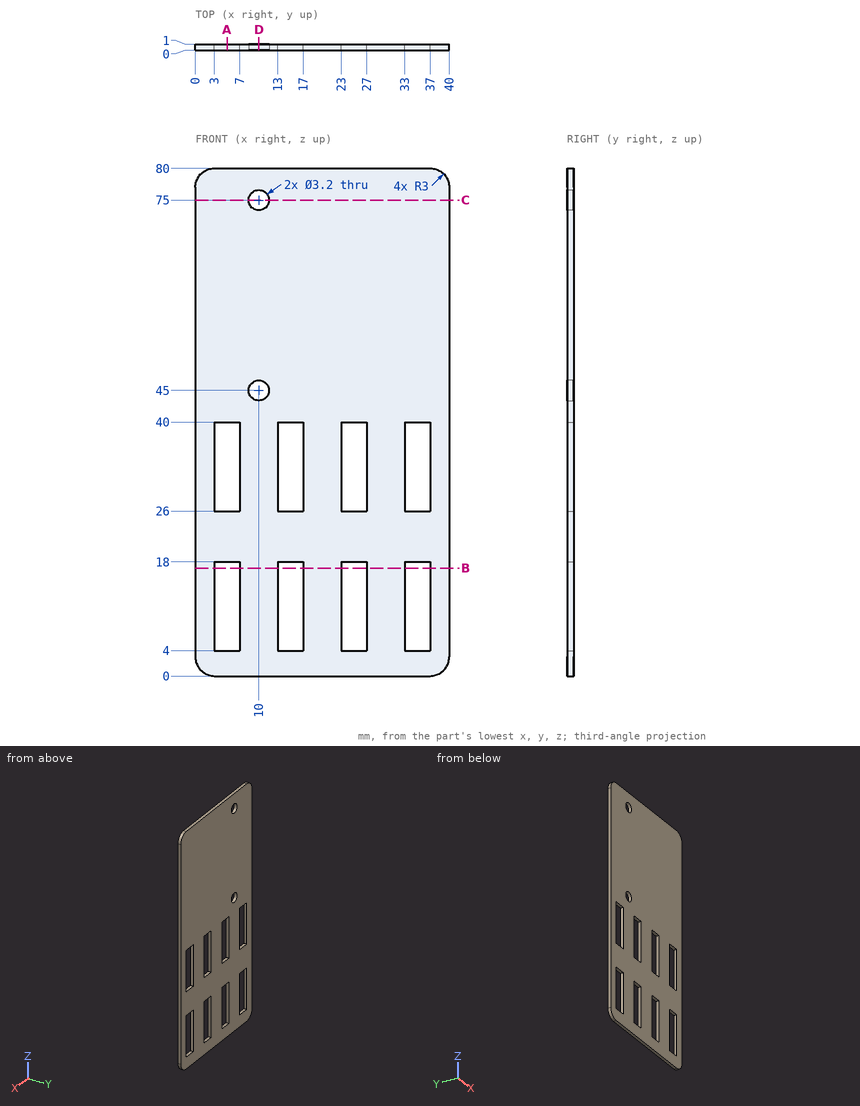
Drawing for the job (mm, zero at the part's lowest x, y, z). Coordinates: 2 decimals unless noted, no trailing zeros. Order: outer loops, then holes, each group sorted by start corner. A loop starts at its lowest first (then second) coordinate and runs counter-clockwise, first axis right, second up. Notation, with made-up numbers: (82, -11.75) -> (110, -11.75) arc R30 ccw to (110, 26.25) -> close; hole circle Ø1 at (26.25, 67.25). An arc over 180 degrees is marked (long way). Answer in a Markdown table with one row per item.
1) Flat gauge pin, fed straight in: P1, Ø3, axis at x = 10, z = 75, coming from the +Y side. Where does the tip first touch, or does it go through?
Check values:
| item | result |
|---|---|
| P1 | through |
2) Drill centre lines: line 1 (Z direction, x = 6, y = 0.4); line 2 (X direction, y = 0.7, z = 10); line 3 (X direction, y = 0.6, z = 75). Where is each one in solid material? Low to high.
Check values:
| item | result |
|---|---|
| line 1 | 0 to 4, 18 to 26, 40 to 80 |
| line 2 | 0 to 3, 7 to 13, 17 to 23, 27 to 33, 37 to 40 |
| line 3 | 0 to 8.4, 11.6 to 40 |
3) Band-saw the part on D-D (x = 10). List the corners of the cut face in (y, z), and give its area (3 significant figures).
Check values:
| item | result |
|---|---|
| outline | (0, 0) -> (1, 0) -> (1, 43.4) -> (0, 43.4) -> close; (0, 46.6) -> (1, 46.6) -> (1, 73.4) -> (0, 73.4) -> close; (0, 76.6) -> (1, 76.6) -> (1, 80) -> (0, 80) -> close |
| area | 73.6 mm2 |
4) Band-saw the part on C-C (z = 75). List the corners of the cut face in (x, y).
Check values:
| item | result |
|---|---|
| outline | (0, 0) -> (8.4, 0) -> (8.4, 1) -> (0, 1) -> close; (11.6, 0) -> (40, 0) -> (40, 1) -> (11.6, 1) -> close |
5) Band-saw the part on B-B (z = 17). List the corners of the cut face in (x, y), and give its area (3 significant figures).
Check values:
| item | result |
|---|---|
| outline | (0, 0) -> (3, 0) -> (3, 1) -> (0, 1) -> close; (7, 0) -> (13, 0) -> (13, 1) -> (7, 1) -> close; (17, 0) -> (23, 0) -> (23, 1) -> (17, 1) -> close; (27, 0) -> (33, 0) -> (33, 1) -> (27, 1) -> close; (37, 0) -> (40, 0) -> (40, 1) -> (37, 1) -> close |
| area | 24.0 mm2 |
6) Band-saw the part on A-A (x = 5). List the corners of the cut face in (y, z), and give its area (3 significant figures).
Check values:
| item | result |
|---|---|
| outline | (0, 0) -> (1, 0) -> (1, 4) -> (0, 4) -> close; (0, 18) -> (1, 18) -> (1, 26) -> (0, 26) -> close; (0, 40) -> (1, 40) -> (1, 80) -> (0, 80) -> close |
| area | 52.0 mm2 |
